Part model, mm, in its own coordinate system. Round coordinates to 2 decimals unless told otherwise and drop trailing zeros. Loops run counter-clockwise (first coordinate to the right, second up) from the corner with the lowest first, then second, coordinate; pieces in that order, holes last. Notation, with made-up numbers: (57, 32) - (85, 32) arc R10 cw to (85, 38) - close; hole circle Ø5 at (-9.75, -22.5). An arc over 180 degrees is marked (long way). Write each question's results on one line, items separated by ' | '. Start each with the question number.
(1) Drill centre lines: L1, parallel to X at y = 2.35, z = 3; L2, parallel to X at y = 3.15, z = 1; L3, parallel to Y at x = 2.75, z = 2.75. Where is each one in solid material? Low to high.
(2) Cut at B-B, the plane z = 1. List the corners of the cut face in (x, y), then the cut area to 3 significant figures.
(3) Cut at A-A, the plane x = 1.1. List the corners of the cut face in (y, z), then the cut area to 3 significant figures.
from build123d import *

# Parameters (mm, degrees)
F1_DEPTH = 4
F5_DEPTH = 25
F8_DEPTH = 25


with BuildPart() as f1:
    # F0 (on Front) → F1 (new body)
    with BuildSketch(Plane.XZ):
        Polygon((2, 6.7082039325), (0, 0), (4, 0), align=None)
    extrude(amount=-F1_DEPTH)

    # F4 (on 3pt) → F5 (cut)
    with BuildSketch(Plane(origin=(0, 0, 0), x_dir=(1, 0, 0), z_dir=(0, -0.9583148475, 0.2857142857))):
        Polygon((4, 0), (2, 7), (0, 0), align=None)
    extrude(amount=F5_DEPTH, mode=Mode.SUBTRACT)

    # F7 (on 3pt) → F8 (cut)
    with BuildSketch(Plane(origin=(0, 3.6734693878, 1.0952169686), x_dir=(1, 0, 0), z_dir=(0, -0.9583148475, -0.2857142857))):
        Polygon((4, -1.1428571429), (2, 5.8571428571), (0, -1.1428571429), align=None)
    extrude(amount=-F8_DEPTH, mode=Mode.SUBTRACT)


solid = f1.part
A:
1) L1: 0.89 to 3.11 | L2: 0.3 to 3.7 | L3: 0.82 to 3.18
2) outline: (0.3, 0.3) - (3.7, 0.3) - (3.7, 3.7) - (0.3, 3.7) - close | area: 11.6 mm2
3) outline: (0, 0) - (4, 0) - (2.9, 3.69) - (1.1, 3.69) - close | area: 10.7 mm2
